```python
from build123d import *

# Parameters (mm, degrees)
SKETCH_1_W          = 20.4
SKETCH_1_H          = 20.4
EXTRUDE_1_DEPTH     = 15.2
SKETCH_2_R          = 9.75
EXTRUDE_2_DEPTH     = 2.5
SKETCH_3_R          = 6.5
EXTRUDE_3_DEPTH     = 0.5
CHAMFER_1_SIZE      = 0.3
CHAMFER_2_SIZE      = 0.3
SKETCH_4_R          = 2.5
EXTRUDE_4_DEPTH     = 10
SKETCH_5_R          = 4.5
EXTRUDE_5_DEPTH     = 0.8
SKETCH_6_R          = 1.5
EXTRUDE_6_DEPTH     = 8
CHAMFER_3_SIZE      = 0.3
CUT_EXTRUDE_1_DEPTH = 1.5
SKETCH_8_R          = 1
CUT_EXTRUDE_2_DEPTH = 6
SKETCH_9_R          = 1.25
CUT_EXTRUDE_3_DEPTH = 1.5
SKETCH_10_R         = 1
CUT_EXTRUDE_4_DEPTH = 4
SKETCH_11_R         = 0.8
CUT_EXTRUDE_5_DEPTH = 1.2
CHAMFER_4_SIZE      = 1.743
CHAMFER_5_SIZE      = 0.3
CUT_EXTRUDE_START   = -9
CUT_EXTRUDE_6_DEPTH = 9
CUT_EXTRUDE_START_2 = -7
CUT_EXTRUDE_7_DEPTH = 7


with BuildPart() as part:
    # 草图1 → 凸台-拉伸1 (new body)
    with BuildSketch(Plane(origin=(0, 0, 0), x_dir=(1, 0, 0), z_dir=(0, 1, 0))):
        Rectangle(SKETCH_1_W, SKETCH_1_H)
    extrude(amount=EXTRUDE_1_DEPTH)

    # 草图2 → 凸台-拉伸2 (add)
    with BuildSketch(Plane(origin=(0, 15.2, 0), x_dir=(1, 0, 0), z_dir=(0, 1, 0))):
        with Locations(Location((0, 0, 0), (0, 0, 270))):
            Circle(SKETCH_2_R)
    extrude(amount=EXTRUDE_2_DEPTH)

    # 草图3 → 凸台-拉伸3 (add)
    with BuildSketch(Plane(origin=(0, 17.7, 0), x_dir=(1, 0, 0), z_dir=(0, 1, 0))):
        with Locations(Location((0, 0, 0), (0, 0, 270))):
            Circle(SKETCH_3_R)
    extrude(amount=EXTRUDE_3_DEPTH)

    # 倒角1
    chamfer_1_edges = [part.edges().sort_by_distance(p)[0] for p in [
        (0, 18.2, -6.5),
    ]]
    chamfer(chamfer_1_edges, length=CHAMFER_1_SIZE)

    # 倒角2
    chamfer_2_edges = [part.edges().sort_by_distance(p)[0] for p in [
        (0, 17.7, -9.75),
    ]]
    chamfer(chamfer_2_edges, length=CHAMFER_2_SIZE)

    # 草图4 → 凸台-拉伸4 (add)
    with BuildSketch(Plane(origin=(0, 18.2, 0), x_dir=(1, 0, 0), z_dir=(0, 1, 0))):
        with Locations(Location((0, 0, 0), (0, 0, 270))):
            Circle(SKETCH_4_R)
    extrude(amount=EXTRUDE_4_DEPTH)

    # 草图5 → 凸台-拉伸5 (add)
    with BuildSketch(Plane.XZ):
        with Locations(Location((0, 0, 0), (0, 0, 270))):
            Circle(SKETCH_5_R)
    extrude(amount=EXTRUDE_5_DEPTH)

    # 草图6 → 凸台-拉伸6 (add)
    with BuildSketch(Plane.XZ.offset(0.8)):
        with Locations(Location((0, 0, 0), (0, 0, 270))):
            Circle(SKETCH_6_R)
    extrude(amount=EXTRUDE_6_DEPTH)

    # 倒角3
    chamfer_3_edges = [part.edges().sort_by_distance(p)[0] for p in [
        (0, -0.8, 4.5),
        (0, -8.8, 1.5),
    ]]
    chamfer(chamfer_3_edges, length=CHAMFER_3_SIZE)

    # 草图7 → 切除-拉伸1 (cut)
    with BuildSketch(Plane.XZ):
        with BuildLine():
            Line((-10.2, 5.8), (-8.5, 5.8))
            ThreePointArc((-8.5, 5.8), (-6.590811691, 6.590811691), (-5.8, 8.5))
            Line((-5.8, 8.5), (-5.8, 10.2))
            Line((-5.8, 10.2), (-10.2, 10.2))
            Line((-10.2, 10.2), (-10.2, 5.8))
        make_face()
        with BuildLine():
            Line((10.2, -10.2), (10.2, -5.8))
            Line((10.2, -5.8), (8.5, -5.8))
            ThreePointArc((8.5, -5.8), (6.590811691, -6.590811691), (5.8, -8.5))
            Line((5.8, -8.5), (5.8, -10.2))
            Line((5.8, -10.2), (10.2, -10.2))
        make_face()
    extrude(amount=-CUT_EXTRUDE_1_DEPTH, mode=Mode.SUBTRACT)

    # 草图8 → 切除-拉伸2 (cut)
    with BuildSketch(Plane(origin=(0, 15.2, 0), x_dir=(1, 0, 0), z_dir=(0, 1, 0))):
        with Locations(Location((-8.131727984, 8.131727984, 0), (0, 0, 270))):
            Circle(SKETCH_8_R)
        with Locations(Location((8.131727984, 8.131727984, 0), (0, 0, 270))):
            Circle(SKETCH_8_R)
        with Locations(Location((8.131727984, -8.131727984, 0), (0, 0, 270))):
            Circle(SKETCH_8_R)
        with Locations(Location((-8.131727984, -8.131727984, 0), (0, 0, 270))):
            Circle(SKETCH_8_R)
    extrude(amount=-CUT_EXTRUDE_2_DEPTH, mode=Mode.SUBTRACT)

    # 草图9 → 切除-拉伸3 (cut)
    with BuildSketch(Plane(origin=(0, 9.2, 0), x_dir=(1, 0, 0), z_dir=(0, 1, 0))):
        with Locations(Location((8.131727984, -8.131727984, 0), (0, 0, 270))):
            Circle(SKETCH_9_R)
        with Locations(Location((8.131727984, 8.131727984, 0), (0, 0, 270))):
            Circle(SKETCH_9_R)
        with Locations(Location((-8.131727984, 8.131727984, 0), (0, 0, 270))):
            Circle(SKETCH_9_R)
        with Locations(Location((-8.131727984, -8.131727984, 0), (0, 0, 270))):
            Circle(SKETCH_9_R)
    extrude(amount=-CUT_EXTRUDE_3_DEPTH, mode=Mode.SUBTRACT)

    # 草图10 → 切除-拉伸4 (cut)
    with BuildSketch(Plane(origin=(0, 18.2, 0), x_dir=(1, 0, 0), z_dir=(0, 1, 0))):
        with Locations(Location((0, -4.9, 0), (0, 0, 270))):
            Circle(SKETCH_10_R)
        with Locations(Location((-4.243524479, 2.45, 0), (0, 0, 270))):
            Circle(SKETCH_10_R)
        with Locations(Location((4.243524479, 2.45, 0), (0, 0, 270))):
            Circle(SKETCH_10_R)
    extrude(amount=-CUT_EXTRUDE_4_DEPTH, mode=Mode.SUBTRACT)

    # 草图11 → 切除-拉伸5 (cut)
    with BuildSketch(Plane(origin=(0, 14.2, 0), x_dir=(1, 0, 0), z_dir=(0, 1, 0))):
        with Locations(Location((0, -4.9, 0), (0, 0, 270))):
            Circle(SKETCH_11_R)
        with Locations(Location((-4.243524479, 2.45, 0), (0, 0, 270))):
            Circle(SKETCH_11_R)
        with Locations(Location((4.243524479, 2.45, 0), (0, 0, 270))):
            Circle(SKETCH_11_R)
    extrude(amount=-CUT_EXTRUDE_5_DEPTH, mode=Mode.SUBTRACT)

    # 倒角4
    chamfer_4_edges = [part.edges().sort_by_distance(p)[0] for p in [
        (-10.2, 7.6, -10.2),
        (10.2, 8.35, -10.2),
        (10.2, 7.6, 10.2),
        (-10.2, 8.35, 10.2),
    ]]
    chamfer(chamfer_4_edges, length=CHAMFER_4_SIZE)

    # 倒角5
    chamfer_5_edges = [part.edges().sort_by_distance(p)[0] for p in [
        (0, 28.2, -2.5),
    ]]
    chamfer(chamfer_5_edges, length=CHAMFER_5_SIZE)

    # 草图12 → 切除-拉伸6 (cut)
    with BuildSketch(Plane(origin=(0, 28.2, 0), x_dir=(1, 0, 0), z_dir=(0, 1, 0)).offset(CUT_EXTRUDE_START)):
        with BuildLine():
            Line((-1.356465997, 2.1), (1.356465997, 2.1))
            ThreePointArc((1.356465997, 2.1), (0, 2.5), (-1.356465997, 2.1))
        make_face()
    extrude(amount=CUT_EXTRUDE_6_DEPTH, mode=Mode.SUBTRACT)

    # 草图13 → 切除-拉伸7 (cut)
    with BuildSketch(Plane.XZ.offset(8.8).offset(CUT_EXTRUDE_START_2)):
        with BuildLine():
            Line((-1.019803903, -1.1), (1.019803903, -1.1))
            ThreePointArc((1.019803903, -1.1), (0, -1.5), (-1.019803903, -1.1))
        make_face()
    extrude(amount=CUT_EXTRUDE_7_DEPTH, mode=Mode.SUBTRACT)


solid = part.part
```
The listing builds one solid part. Answer for the finished solid, in the listing's coordinates (mm). A direction names the side the tool comes from. Round coordinates to 2 decimals unless told otherwise and drop trailing zeros. Loops run counter-clockwise (first coordinate to the right, second up) from the corner with the lowest first, then second, coordinate; pieces in that order, holes last.
Q1. Find the intervals of material crossed by line 1 (Z direction, x = 8, y = 11); line 2 (X direction, y = 13.5, z = -2.45); line 3 (X direction, y = 15.7, z = -2.45), in increasing order.
Q2. Section A-A, the plane y = 1 is taken. Determine the outline of the cut face in (x, z).
Q3. Given pin 1 Ø2 at (x, z) = (5.5, 1) entering from -Y; pin 2 Ø0.8 at (x, z) = (-8.5, 8) entering from -Y; pin 3 Ø6 at (y, z) = (-4.5, -1) entering from -X; pin 4 Ø12 at (x, y) = (-1, 16.5) entering from +Z, each flat-ended and moving along its own axis, determine where each tip first touches the part or whether it passes through.
Q4. Section B-B, the plane y = 10 is taken. Determine the outline of the cut face in (x, z).
Q5. For a pull along Y with two mould halves and no side action, classify faces 4 (the face through (8, 1.5, -8)), 5 (the face through (7.37, 8.46, 7.14)), 6 (the face through (-8.09, 12.24, -9.13)) as released by +Y, released by -Y, zero draft, split by the parting line, or undercut.
Q6. Which of the six approach directions +Z, -Z, +X, -X, +Y, -Y give full straight-line access (tool end or side, diameter ignored) to faces 1 (the face through (-9, 1, 5.8)), 2 (the face through (4, 13, -2)), 3 (the face through (0.07, -4.6, 1.5))?
Q7. Section C-C, the plane y = 20 is taken. Determine the outline of the cut face in (x, z).
Completed:
1. line 1: z = -10.2 to -9.12, -7.14 to 7.14, 9.12 to 10.2
1. line 2: x = -10.2 to -5.04, -3.44 to 3.44, 5.04 to 10.2
1. line 3: x = -9.44 to -5.24, -3.24 to 3.24, 5.24 to 9.44
2. outline: (-10.2, -8.46) - (-8.46, -10.2) - (5.8, -10.2) - (5.8, -8.5) arc R2.7 cw to (8.5, -5.8) - (10.2, -5.8) - (10.2, 8.46) - (8.46, 10.2) - (-5.8, 10.2) - (-5.8, 8.5) arc R2.7 cw to (-8.5, 5.8) - (-10.2, 5.8) - close
3. pin 1: stops at y = 0
3. pin 2: stops at y = 1.5
3. pin 3: stops at x = -1.5
3. pin 4: stops at z = 10.2
4. outline: (-10.2, -8.46) - (-8.46, -10.2) - (8.46, -10.2) - (10.2, -8.46) - (10.2, 8.46) - (8.46, 10.2) - (-8.46, 10.2) - (-10.2, 8.46) - close; hole circle Ø2 at (-8.13, -8.13); hole circle Ø2 at (-8.13, 8.13); hole circle Ø2 at (8.13, -8.13); hole circle Ø2 at (8.13, 8.13)
5. face 4: released by -Y
5. face 5: undercut
5. face 6: zero draft
6. face 1: +Z, -X, -Y
6. face 2: +Y
6. face 3: -Y
7. outline: (-1.36, -2.1) - (1.36, -2.1) arc R2.5 ccw (long way) to start
